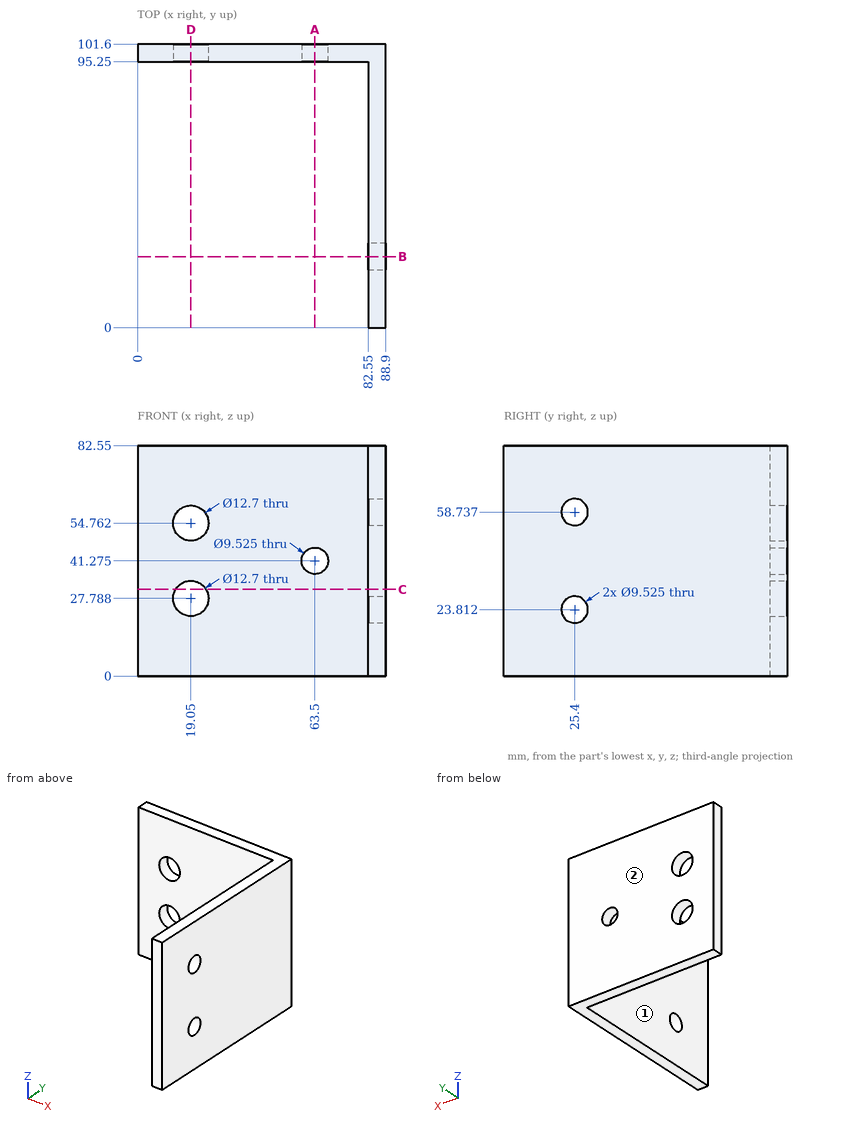
Could you check a few things on this drawing? It's one solid part, dimensions in mm from its lowest x, y, z. A direction names the side the tool comes from. Coordinates: 2 decimals unless noted, no trailing zeros. Write each loop counter-clockwise with the first axis right and the second up, starting at its lowest first coordinate (ties: lowest second). Pieces come first, ordered by that corner, then holes.
1) If we section it at B-B (y = 25.4): Count the separate pieces of the cut face and the enclosed holes in it, plus the area to 3 significant figures.
Filled in:
separate pieces: 3
enclosed holes: 0
area: 403 mm2
2) If I drill on line 1 (Z direction, x = 19, y = 97); line 2 (Z direction, x = 63.5, y = 98.5); line 3 (Y direction, x = 72, z = 19.5), over which ranges is the centre line in solid material (lowest first)?
Filled in:
line 1: z = 0 to 21.44, 34.14 to 48.41, 61.11 to 82.55
line 2: z = 0 to 36.51, 46.04 to 82.55
line 3: y = 95.25 to 101.6
3) If we section it at D-D (x = 19.05): List the corners of the cut face in (y, z) for me, plus the area to 3 significant figures.
Filled in:
outline: (95.25, 0) - (101.6, 0) - (101.6, 21.44) - (95.25, 21.44) - close; (95.25, 34.14) - (101.6, 34.14) - (101.6, 48.41) - (95.25, 48.41) - close; (95.25, 61.11) - (101.6, 61.11) - (101.6, 82.55) - (95.25, 82.55) - close
area: 363 mm2
4) If we section it at C-C (z = 31): List the corners of the cut face in (x, y) for me, plus the area to 3 significant figures.
Filled in:
outline: (0, 95.25) - (13.57, 95.25) - (13.57, 101.6) - (0, 101.6) - close; (24.53, 95.25) - (82.55, 95.25) - (82.55, 0) - (88.9, 0) - (88.9, 101.6) - (24.53, 101.6) - close
area: 1,100 mm2
5) I'm going to push flat-ended pins straight in: pin 1 (25 mm diameter, centred on x = 51.5, z = 51.5, fed in from -Y); pin 2 (12.5 mm diameter, centred on y = 25.4, z = 23.81, fed in from +X); pin 3 (3 mm diameter, centred on y = 77, z = 22.5, fed in from -X). Where does each tip first touch, or does it pass through?
Filled in:
pin 1: stops at y = 95.25
pin 2: stops at x = 88.9
pin 3: stops at x = 82.55
6) If we section it at A-A (x = 63.5): List the corners of the cut face in (y, z) for me, plus the area to 3 significant figures.
Filled in:
outline: (95.25, 0) - (101.6, 0) - (101.6, 36.51) - (95.25, 36.51) - close; (95.25, 46.04) - (101.6, 46.04) - (101.6, 82.55) - (95.25, 82.55) - close
area: 464 mm2
7) Which directions (+Z, -Z, +X, -X, +Y, -Y) give clear straight access to the entire face, cutting with the end or side of a thin tool? Please do the marked faces 1 and 2.
Filled in:
face 1: +Z, -Z, -X, -Y
face 2: +Z, -Z, +X, -X, +Y
